Drawing for the job (mm, zero at the part's lowest x, y, z). A direction names the side the tool comes from. Round coordinates to 2 decimals unless told otherwise and drop trailing zeros. Loops run counter-clockwise (first coordinate to the right, second up) from the corner with the lowest first, then second, coordinate; pieces in that order, holes last. Notation, with made-up numbers: (-25.5, 76) -> (21.5, 76) arc R13 cw to (21.5, 99) -> close; hole circle Ø10 at (70.25, -3). An arc over 180 degrees is marked (long way). Put each result on its own line as item: value. Start each with the question number.
Item 1: Cut at D-D, the plane y = 0.75. List the corners of the cut face in (x, z) (1 decimal).
Item 2: Cut at A-A, the plane y = 2.5. List the corners of the cut face in (x, z) (1 decimal).
Item 3: Cut at C-C, the plane z = 2.25. List the corners of the cut face in (x, y).
Item 4: Cut at B-B, the plane x = 25.5. List the corners of the cut face in (y, z), plus the area to 3 significant figures.
Item 5: Drill centre lines: probe 1 along Y at (x, z) = (2.5, 7.7); probe 2 along X at (y, z) = (2.7, 7.75); probe 3 along Z at (x, y) = (5, 3.1). Where is each one in solid material? Low to high. Write a range as [from, to].
Item 6: Tool access for the marked faces 1, 2 and 3: list every direction of +Z, -Z, +X, -X, +Y, -Y with a clear straight run to the whole face (end or side of a thin tool).
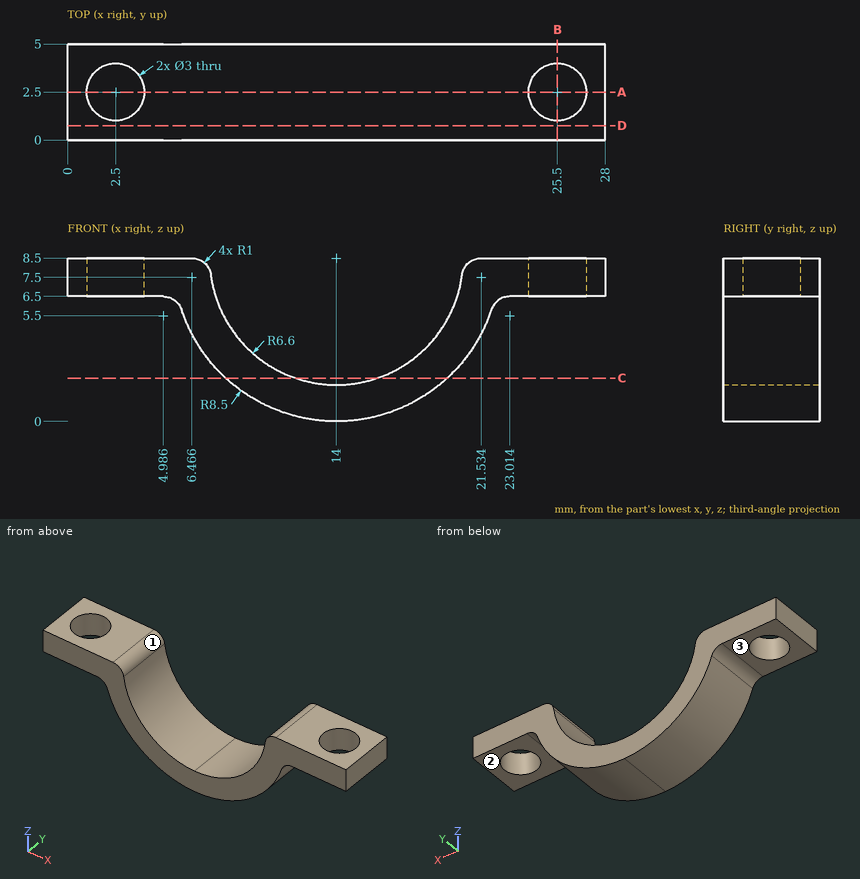
Reply:
1. outline: (0, 6.5) -> (5, 6.5) arc R1 cw to (5.9, 5.8) arc R8.5 ccw to (22.1, 5.8) arc R1 cw to (23, 6.5) -> (28, 6.5) -> (28, 8.5) -> (21.5, 8.5) arc R1 ccw to (20.5, 7.6) arc R6.6 cw to (7.5, 7.6) arc R1 ccw to (6.5, 8.5) -> (0, 8.5) -> close
2. outline: (0, 6.5) -> (1, 6.5) -> (1, 8.5) -> (0, 8.5) -> close; (4, 6.5) -> (5, 6.5) arc R1 cw to (5.9, 5.8) arc R8.5 ccw to (22.1, 5.8) arc R1 cw to (23, 6.5) -> (24, 6.5) -> (24, 8.5) -> (21.5, 8.5) arc R1 ccw to (20.5, 7.6) arc R6.6 cw to (7.5, 7.6) arc R1 ccw to (6.5, 8.5) -> (4, 8.5) -> close; (27, 6.5) -> (28, 6.5) -> (28, 8.5) -> (27, 8.5) -> close
3. outline: (8.24, 0) -> (11.88, 0) -> (11.88, 5) -> (8.24, 5) -> close; (16.12, 0) -> (19.76, 0) -> (19.76, 5) -> (16.12, 5) -> close
4. outline: (0, 6.5) -> (1, 6.5) -> (1, 8.5) -> (0, 8.5) -> close; (4, 6.5) -> (5, 6.5) -> (5, 8.5) -> (4, 8.5) -> close
4. area: 4.00 mm^2
5. probe 1: y = [0, 1], [4, 5]
5. probe 2: x = [0, 1.01], [3.99, 7.43], [20.57, 24.01], [26.99, 28]
5. probe 3: z = [6.5, 8.5]
6. face 1: +Z, +Y, -Y
6. face 2: -Z, +X, +Y, -Y
6. face 3: -Z, -X, +Y, -Y
